Read the model definition and answer for the solid it produces. Units are mm, in the model's axes. Round coordinates to 2 decimals unless told otherwise and drop trailing zeros. Order: outer loops, then holes, each group sorted by start corner. A loop starts at its lowest first (then second) coordinate and runs counter-clockwise, first axis right, second up. Notation, with made-up numbers: (-34, -29.75) -> (13, -29.75) arc R20 cw to (13, 4.25) -> close; hole circle Ø11 at (71.25, 0.5). An arc over 180 degrees is marked (long way). One line per item, written item: value. Start each with the question number.
1. Section C-C (z = 2.25) is taken. State how many separate pieces and enclosed holes the cut face has, then the cut area to 3 significant figures.
2. Flat-ended cylindrical pins translate along their axes: pin 1 Ø6 at (x, y) = (-84, 26.5) entering from -Z; pin 2 Ø1.5 at (y, z) = (37.5, 1) entering from -X; pin 3 Ø0.9 at (y, z) = (36, 2) entering from -X; pin 4 Ø1.5 at (x, z) = (-75, 1) entering from -Y. Find the tip coordinate at first contact, or state that the pin passes through.
3. Consider line 1 (X direction, y = -21.5, z = 1.4); line 2 (Y direction, x = 5.5, z = 2.25); line 3 (Y direction, x = -46, z = 0.55). Determine where each line is inside the solid, lowest interval first.
4. Section B-B (x = -1) is taken. Give the vertices of the cut face in (y, z).
5. Section A-A (x = -65.5) is taken. Give the vertices of the cut face in (y, z).
from build123d import *

# Parameters (mm, degrees)
SKETCH1_W           = 3
SKETCH1_H           = 12.7
SKETCH1_W_2         = 6.35
SKETCH1_H_2         = 3
SKETCH1_W_3         = 19.05
SKETCH1_W_4         = 11
SKETCH1_H_3         = 13
BOSS_EXTRUDE1_DEPTH = 3


with BuildPart() as part:
    # Sketch1 → Boss-Extrude1 (new body)
    with BuildSketch(Plane.XY):
        with BuildLine():
            Line((50.8, 31.75), (50.8, -31.75))
            Line((50.8, -31.75), (27.1653, -31.75))
            Line((27.1653, -31.75), (27.1653, -26.67))
            Line((27.1653, -26.67), (29.5275, -26.67))
            Line((29.5275, -26.67), (29.5275, -21.59))
            Line((29.5275, -21.59), (21.2725, -21.59))
            Line((21.2725, -21.59), (21.2725, -26.67))
            Line((21.2725, -26.67), (23.6347, -26.67))
            Line((23.6347, -26.67), (23.6347, -31.75))
            Line((23.6347, -31.75), (9.525, -31.75))
            Line((9.525, -31.75), (9.525, -34.75))
            Line((9.525, -34.75), (-9.525, -34.75))
            Line((-9.525, -34.75), (-9.525, -31.75))
            Line((-9.525, -31.75), (-23.6347, -31.75))
            Line((-23.6347, -31.75), (-23.6347, -26.67))
            Line((-23.6347, -26.67), (-21.2725, -26.67))
            Line((-21.2725, -26.67), (-21.2725, -21.59))
            Line((-21.2725, -21.59), (-29.5275, -21.59))
            Line((-29.5275, -21.59), (-29.5275, -26.67))
            Line((-29.5275, -26.67), (-27.1653, -26.67))
            Line((-27.1653, -26.67), (-27.1653, -31.75))
            Line((-27.1653, -31.75), (-41.275, -31.75))
            Line((-41.275, -31.75), (-41.275, -34.75))
            Line((-41.275, -34.75), (-60.325, -34.75))
            Line((-60.325, -34.75), (-60.325, -31.75))
            Line((-60.325, -31.75), (-74.4347, -31.75))
            Line((-74.4347, -31.75), (-74.4347, -26.67))
            Line((-74.4347, -26.67), (-72.0725, -26.67))
            Line((-72.0725, -26.67), (-72.0725, -21.59))
            Line((-72.0725, -21.59), (-80.3275, -21.59))
            Line((-80.3275, -21.59), (-80.3275, -26.67))
            Line((-80.3275, -26.67), (-77.9653, -26.67))
            Line((-77.9653, -26.67), (-77.9653, -31.75))
            Line((-77.9653, -31.75), (-90.25, -31.75))
            Line((-90.25, -31.75), (-90.25, -18.75))
            Line((-90.25, -18.75), (-101.25, -18.75))
            Line((-101.25, -18.75), (-101.25, -31.75))
            Line((-101.25, -31.75), (-114.3, -31.75))
            Line((-114.3, -31.75), (-114.3, 12.7))
            add(Edge.make_bspline(
                [(-114.3, 12.7), (-114.446449762, 40.172975461), (-95.462376933, 57.15)],
                knots=[0, 0, 0, 1, 1, 1], degree=2))
            Line((-95.462376933, 57.15), (50.8, 57.15))
            Line((50.8, 57.15), (50.8, 31.75))
        make_face()
        with BuildLine():
            Line((33.200035124, 7.62), (33.200035124, -5.08))
            ThreePointArc((33.200035124, -5.08), (25.580035124, -12.7), (17.960035124, -5.08))
            Line((17.960035124, -5.08), (17.960035124, 7.62))
            ThreePointArc((17.960035124, 7.62), (25.580035124, 15.24), (33.200035124, 7.62))
        make_face(mode=Mode.SUBTRACT)
        with Locations((44.22, 38.1)):
            Rectangle(SKETCH1_W, SKETCH1_H, mode=Mode.SUBTRACT)
        with BuildLine():
            Line((10.340035124, 7.62), (10.340035124, -5.08))
            ThreePointArc((10.340035124, -5.08), (2.720035124, -12.7), (-4.899964876, -5.08))
            Line((-4.899964876, -5.08), (-4.899964876, 7.62))
            ThreePointArc((-4.899964876, 7.62), (2.720035124, 15.24), (10.340035124, 7.62))
        make_face(mode=Mode.SUBTRACT)
        with BuildLine():
            Line((-12.519964876, 7.62), (-12.519964876, -5.08))
            ThreePointArc((-12.519964876, -5.08), (-20.139964876, -12.7), (-27.759964876, -5.08))
            Line((-27.759964876, -5.08), (-27.759964876, 7.62))
            ThreePointArc((-27.759964876, 7.62), (-20.139964876, 15.24), (-12.519964876, 7.62))
        make_face(mode=Mode.SUBTRACT)
        with Locations((44.22, 0)):
            Rectangle(SKETCH1_W, SKETCH1_H, mode=Mode.SUBTRACT)
        with BuildLine():
            Line((-35.379964876, 7.62), (-35.379964876, -5.08))
            ThreePointArc((-35.379964876, -5.08), (-42.999964876, -12.7), (-50.619964876, -5.08))
            Line((-50.619964876, -5.08), (-50.619964876, 7.62))
            ThreePointArc((-50.619964876, 7.62), (-42.999964876, 15.24), (-35.379964876, 7.62))
        make_face(mode=Mode.SUBTRACT)
        with BuildLine():
            Line((-58.239964876, 7.62), (-58.239964876, -5.08))
            ThreePointArc((-58.239964876, -5.08), (-65.859964876, -12.7), (-73.479964876, -5.08))
            Line((-73.479964876, -5.08), (-73.479964876, 7.62))
            ThreePointArc((-73.479964876, 7.62), (-65.859964876, 15.24), (-58.239964876, 7.62))
        make_face(mode=Mode.SUBTRACT)
        with BuildLine():
            Line((33.200035124, 44.45), (33.200035124, 31.75))
            ThreePointArc((33.200035124, 31.75), (25.580035124, 24.13), (17.960035124, 31.75))
            Line((17.960035124, 31.75), (17.960035124, 44.45))
            ThreePointArc((17.960035124, 44.45), (25.580035124, 52.07), (33.200035124, 44.45))
        make_face(mode=Mode.SUBTRACT)
        with BuildLine():
            Line((10.340035124, 44.45), (10.340035124, 31.75))
            ThreePointArc((10.340035124, 31.75), (2.720035124, 24.13), (-4.899964876, 31.75))
            Line((-4.899964876, 31.75), (-4.899964876, 44.45))
            ThreePointArc((-4.899964876, 44.45), (2.720035124, 52.07), (10.340035124, 44.45))
        make_face(mode=Mode.SUBTRACT)
        with BuildLine():
            Line((-12.519964876, 44.45), (-12.519964876, 31.75))
            ThreePointArc((-12.519964876, 31.75), (-20.139964876, 24.13), (-27.759964876, 31.75))
            Line((-27.759964876, 31.75), (-27.759964876, 44.45))
            ThreePointArc((-27.759964876, 44.45), (-20.139964876, 52.07), (-12.519964876, 44.45))
        make_face(mode=Mode.SUBTRACT)
        with BuildLine():
            Line((-35.379964876, 44.45), (-35.379964876, 31.75))
            ThreePointArc((-35.379964876, 31.75), (-42.999964876, 24.13), (-50.619964876, 31.75))
            Line((-50.619964876, 31.75), (-50.619964876, 44.45))
            ThreePointArc((-50.619964876, 44.45), (-42.999964876, 52.07), (-35.379964876, 44.45))
        make_face(mode=Mode.SUBTRACT)
        with BuildLine():
            Line((-58.239964876, 44.45), (-58.239964876, 31.75))
            ThreePointArc((-58.239964876, 31.75), (-65.859964876, 24.13), (-73.479964876, 31.75))
            Line((-73.479964876, 31.75), (-73.479964876, 44.45))
            ThreePointArc((-73.479964876, 44.45), (-65.859964876, 52.07), (-58.239964876, 44.45))
        make_face(mode=Mode.SUBTRACT)
        Polygon((-108.570127811, 2.130538697), (-108.570127811, 8.521708079), (-106.677281982, 21.226947449), (-101.67507942, 21.226947449), (-88.964755701, 21.226947449), (-88.964755701, -6.382139969), (-108.570127811, -6.382139969), align=None, mode=Mode.SUBTRACT)
        with Locations((-88.193493425, 41.3464095)):
            Rectangle(SKETCH1_W_2, SKETCH1_H_2, mode=Mode.SUBTRACT)
        with Locations((23.495, 20.550240793)):
            Rectangle(SKETCH1_W_3, SKETCH1_H_2, mode=Mode.SUBTRACT)
        with Locations((-8.255, 20.550240793)):
            Rectangle(SKETCH1_W_3, SKETCH1_H_2, mode=Mode.SUBTRACT)
        with Locations((-0.113307165, -25.25)):
            Rectangle(SKETCH1_W_4, SKETCH1_H_3, mode=Mode.SUBTRACT)
    extrude(amount=BOSS_EXTRUDE1_DEPTH)


solid = part.part
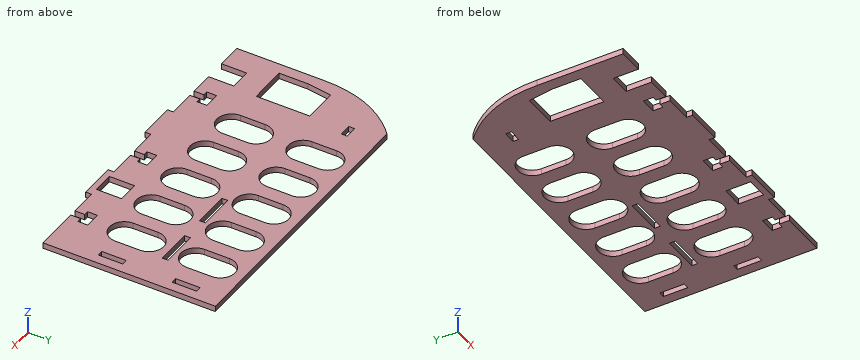
Answer:
1. separate pieces: 1
1. enclosed holes: 17
1. area: 9,580 mm^2
2. pin 1: z = 0
2. pin 2: x = -109.99
2. pin 3: x = -110.46
2. pin 4: y = -31.75
3. line 1: -114.3 to -101.25, -90.25 to -5.61, 5.39 to 50.8
3. line 2: -34.75 to -12.17, 14.71 to 24.66, 51.54 to 57.15
3. line 3: -34.75 to -12.08, 14.62 to 24.75, 51.45 to 57.15
4. outline: (-34.75, 0) -> (-31.75, 0) -> (-31.75, 3) -> (-34.75, 3) -> close; (-18.75, 0) -> (-11.73, 0) -> (-11.73, 3) -> (-18.75, 3) -> close; (14.27, 0) -> (19.05, 0) -> (19.05, 3) -> (14.27, 3) -> close; (22.05, 0) -> (25.1, 0) -> (25.1, 3) -> (22.05, 3) -> close; (51.1, 0) -> (57.15, 0) -> (57.15, 3) -> (51.1, 3) -> close
5. outline: (-31.75, 0) -> (-12.69, 0) -> (-12.69, 3) -> (-31.75, 3) -> close; (15.23, 0) -> (24.14, 0) -> (24.14, 3) -> (15.23, 3) -> close; (52.06, 0) -> (57.15, 0) -> (57.15, 3) -> (52.06, 3) -> close
